Design review of the part shown in the three views and the two pictorial views. Dimensions are in mm from the part's minimum x, y and z. Give positions to 0.01 mm unless a question says otherwise; leave off trailing zeros. Order: outer loops, then holes, each group sorted by start corner. A loop starts at its lowest first (then second) coordinate and runs counter-clockwise, first axis right, second up.
Item 1: Consider section C-C (z = 13.25). Give the boundary of the cut face in (x, y) (3 decimals).
Item 2: Consider section B-B (x = 145.5). Give the boundary of the cut face in (y, z) (3 decimals), plus the area to 3 significant figures.
Item 3: Consider section A-A (y = 477). Give the boundary of the cut face in (x, z).
Item 4: For probe 1 along Y at (x, z) = (803.5, 15.25) (3 decimals); probe 2 along X at (y, z) = (681.5, 11), list the stretches that pass through material, from the lowest coordinate up.
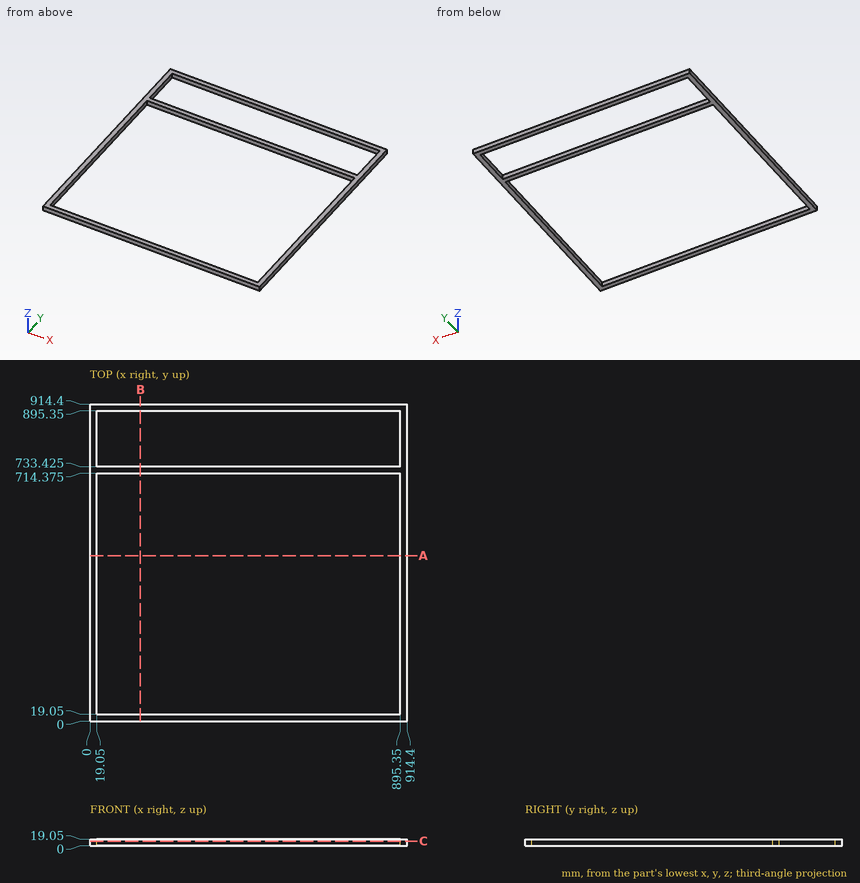
Resolved:
1. outline: (0, 0) - (914.4, 0) - (914.4, 914.4) - (0, 914.4) - close; hole (19.05, 19.05) - (895.35, 19.05) - (895.35, 714.375) - (19.05, 714.375) - close; hole (19.05, 733.425) - (895.35, 733.425) - (895.35, 895.35) - (19.05, 895.35) - close
2. outline: (0, 0) - (19.05, 0) - (19.05, 19.05) - (0, 19.05) - close; (714.375, 0) - (733.425, 0) - (733.425, 19.05) - (714.375, 19.05) - close; (895.35, 0) - (914.4, 0) - (914.4, 19.05) - (895.35, 19.05) - close
2. area: 1,090 mm2
3. outline: (0, 0) - (19.05, 0) - (19.05, 19.05) - (0, 19.05) - close; (895.35, 0) - (914.4, 0) - (914.4, 19.05) - (895.35, 19.05) - close
4. probe 1: y = 0 to 19.05, 714.375 to 733.425, 895.35 to 914.4
4. probe 2: x = 0 to 19.05, 895.35 to 914.4
